```python
from build123d import *

# Parameters (mm, degrees)
SKETCH014_R             = 11
PAD013_DEPTH            = 2
SKETCH015_R             = 6.5
POCKET005_DEPTH         = 1
SKETCH016_R             = 11
SKETCH016_R_2           = 10.5
PAD014_DEPTH            = 24
SKETCH017_R             = 2.25
POCKET006_DEPTH         = 12
BODY009_PLACEMENT_ANGLE = 180


with BuildPart() as part:
    # Sketch014 → Pad013 (new body)
    with BuildSketch(Plane.XY):
        Circle(SKETCH014_R)
    extrude(amount=PAD013_DEPTH)

    # Sketch015 (on Face3 of Pad013) → Pocket005 (cut)
    with BuildSketch(Plane.XY.offset(2)):
        Circle(SKETCH015_R)
    extrude(amount=-POCKET005_DEPTH, mode=Mode.SUBTRACT)

    # Sketch016 (on Face3 of Pocket005) → Pad014 (join)
    with BuildSketch(Plane.XY.offset(2)):
        Circle(SKETCH016_R)
        Circle(SKETCH016_R_2, mode=Mode.SUBTRACT)
    extrude(amount=PAD014_DEPTH)

    # Sketch017 → Pocket006 (cut, symmetric)
    with BuildSketch(Plane.XZ):
        with Locations((0, 15)):
            Circle(SKETCH017_R)
    extrude(amount=POCKET006_DEPTH, both=True, mode=Mode.SUBTRACT)


with BuildPart() as part_1:
    # Body009 placement: moved
    add(part.part.moved(Location((0, 0, 30))).rotate(Axis((0, 0, 30), (1, 0, 0)), BODY009_PLACEMENT_ANGLE))


solid = part_1.part
```
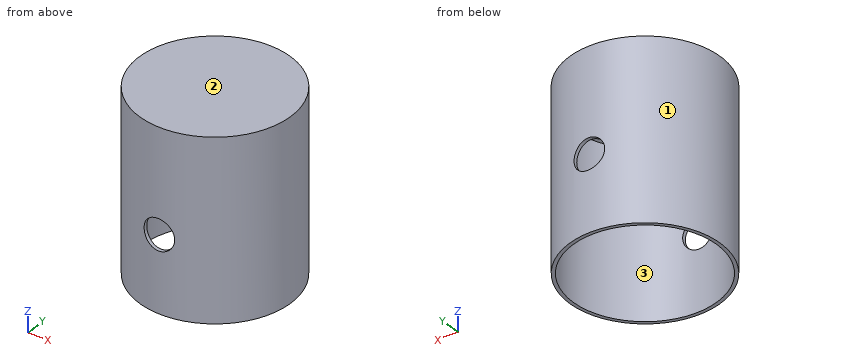
Can you work these out from the model? Positions are in its coordinate system, mm. Face numbers are marked on the shaded views. Round coordinates to 2 decimals unless told otherwise and drop trailing zeros. Loops run counter-clockwise (first coordinate to the right, second up) from the corner with the lowest first, then second, coordinate; pieces in that order, holes last. Notation, with made-up numbers: M 40,80.5 L 54,80.5 A24 cw 54,100.5 Z; hole C 62,37 d6. An arc over 180 degrees is marked long. Answer as a JSON object with one key per item and string values. Group by question number.
Q1. Imagine slicing it at C-C, the plane z = 15. Please give me the cut outline in (x, y).
Q2. Imagine slicing it at D-D, the plane x = 9.25. Please give me the cut outline in (y, z).
Q3. Imagine slicing it at B-B, the plane y = 0. Please give me the cut outline in (x, z), then the cut area to 3 significant figures.
Q4. Will these pins go through, and if not, where does the flat tip stop? pin 1 (1.5 mm diameter, centred on y = 7.5, z = 18, fed in from -X); pin 2 (5 mm diameter, centred on x = -6, y = 0, fed in from -Z); pin 3 (4 mm diameter, centred on y = -4.5, z = 26.5, fed in from -X).
Q5. We'd pull the mould along Y, two halves only. Please class the marked faces 1, 2 and 3: +Y half, -Y half, draft (parallel to the pull), parting line (faces both ways), or undercut.
Q6. Imagine slicing it at A-A, the plane x = 0. Please give me the cut outline in (y, z).
Q7. Please list where these lines run through material, in increasing order: L1, parallel to X at y = 0, z = 28.7; L2, parallel to X at y = 0, z = 16.25.
Findings:
{
 "1": {"outline": "M -2.25,-10.77 L -2.25,-10.26 A10.5 cw -2.25,10.26 L -2.25,10.77 A11 ccw Z; M 2.25,-10.77 A11 ccw 2.25,10.77 L 2.25,10.26 A10.5 cw 2.25,-10.26 Z"},
 "2": {"outline": "M -5.95,4 L -4.97,4 L -4.97,28 L 4.97,28 L 4.97,4 L 5.95,4 L 5.95,30 L -5.95,30 Z"},
 "3": {"outline": "M -11,4 L -10.5,4 L -10.5,28 L -6.5,28 L -6.5,29 L 6.5,29 L 6.5,28 L 10.5,28 L 10.5,4 L 11,4 L 11,30 L -11,30 Z", "area": "55.0 mm2"},
 "4": {"pin 1": "stops at x = -8.69", "pin 2": "stops at z = 28", "pin 3": "stops at x = -10.71"},
 "5": {"face 1": "parting line", "face 2": "draft", "face 3": "undercut"},
 "6": {"outline": "M -11,4 L -10.5,4 L -10.5,12.75 L -11,12.75 Z; M -11,17.25 L -10.5,17.25 L -10.5,28 L -6.5,28 L -6.5,29 L 6.5,29 L 6.5,28 L 10.5,28 L 10.5,17.25 L 11,17.25 L 11,30 L -11,30 Z; M 10.5,4 L 11,4 L 11,12.75 L 10.5,12.75 Z"},
 "7": {"L1": "x = -11 to -6.5, 6.5 to 11", "L2": "x = -11 to -10.5, 10.5 to 11"}
}
